from build123d import *

# Parameters (mm, degrees)
SKETCH_2_R          = 3
SKETCH_2_R_2        = 1.5
SKETCH_2_R_3        = 2.5
EXTRUDE_1_DEPTH     = 3
EXTRUDE_2_DEPTH     = 196
SKETCH_5_R          = 8
CUT_EXTRUDE_1_DEPTH = 10
SKETCH_6_R          = 4.05
CUT_EXTRUDE_2_DEPTH = 10
SKETCH_8_R          = 40
EXTRUDE_3_DEPTH     = 3
EXTRUDE_START       = -61
EXTRUDE_4_DEPTH     = 64
EXTRUDE_5_DEPTH     = 3
EXTRUDE_START_2     = -3
EXTRUDE_14_DEPTH    = 3
EXTRUDE_15_DEPTH    = 3
SKETCH_16_R         = 40
EXTRUDE_16_DEPTH    = 3
CUT_EXTRUDE_START   = -20
CUT_EXTRUDE_5_DEPTH = 20
CUT_EXTRUDE_6_DEPTH = 20
CUT_EXTRUDE_7_DEPTH = 3
FILLET_3_R          = 3
FILLET_4_R          = 3
FILLET_5_R          = 3
FILLET_6_R          = 3
SKETCH_22_R         = 7.75
CUT_EXTRUDE_8_DEPTH = 10
SKETCH_23_R         = 4.05
CUT_EXTRUDE_9_DEPTH = 10


# Some blends are built 0.0001 mm under size
with BuildPart() as part:
    # Sketch 2 → Extrude 1 (new body)
    with BuildSketch(Plane(origin=(0, 0, 0), x_dir=(0, 0, -1), z_dir=(1, 0, 0))):
        with BuildLine():
            Line((138.514809283, 84.200667909), (-11.70063651, 38.25042621))
            ThreePointArc((-11.70063651, 38.25042621), (-39.560188627, -5.915359313), (0, -40))
            Line((0, -40), (16.710190716, -40))
            Line((16.710190716, -40), (156.071648789, 40.329376559))
            Line((156.071648789, 40.329376559), (156.071648789, 43.792069046))
            ThreePointArc((156.071648789, 43.792069046), (165.334026038, 71.834783727), (138.514809283, 84.200667909))
        make_face()
        Circle(SKETCH_2_R, mode=Mode.SUBTRACT)
        with Locations((145, 70)):
            Circle(SKETCH_2_R_2, mode=Mode.SUBTRACT)
        with Locations((138, 63)):
            Circle(SKETCH_2_R_2, mode=Mode.SUBTRACT)
        with Locations((145, 56)):
            Circle(SKETCH_2_R_2, mode=Mode.SUBTRACT)
        with Locations((145, 63)):
            Circle(SKETCH_2_R_3, mode=Mode.SUBTRACT)
        with Locations((152, 63)):
            Circle(SKETCH_2_R_2, mode=Mode.SUBTRACT)
    extrude_1 = extrude(amount=EXTRUDE_1_DEPTH)

    # Sketch 4 → Extrude 2 (add)
    with BuildSketch(Plane(origin=(3, 0, 0), x_dir=(0, 0, -1), z_dir=(1, 0, 0))):
        with BuildLine():
            Line((0, -40), (16.710190716, -40))
            Line((16.710190716, -40), (156.071648789, 40.329376559))
            Line((156.071648789, 40.329376559), (156.071648789, 43.792069046))
            Line((156.071648789, 43.792069046), (19.975563357, -34.655113166))
            ThreePointArc((19.975563357, -34.655113166), (10.339136167, -38.640681455), (0, -40))
        make_face()
    extrude(amount=EXTRUDE_2_DEPTH)

    # Mirror 2: Extrude 1 across plane
    add(extrude_1.mirror(Plane(origin=(101, 0, 0), x_dir=(0, 0, 1), z_dir=(1, 0, 0))))

    # Sketch 5 → Cut-Extrude 1 (cut)
    with BuildSketch(Plane(origin=(202, 0, 0), x_dir=(0, 0, -1), z_dir=(1, 0, 0))):
        Circle(SKETCH_5_R)
    extrude(amount=-CUT_EXTRUDE_1_DEPTH, mode=Mode.SUBTRACT)

    # Sketch 6 → Cut-Extrude 2 (cut)
    with BuildSketch(Plane.ZY):
        Circle(SKETCH_6_R)
    extrude(amount=-CUT_EXTRUDE_2_DEPTH, mode=Mode.SUBTRACT)

    # Sketch 9 → Extrude 4 (add)
    with BuildSketch(Plane(origin=(251, 0, 0), x_dir=(0, 0, -1), z_dir=(1, 0, 0)).offset(EXTRUDE_START)):
        with BuildLine():
            Line((0, -40), (16.710190716, -40))
            Line((16.710190716, -40), (53.747942483, -18.651059269))
            Line((53.747942483, -18.651059269), (52.249775231, -16.051925781))
            Line((52.249775231, -16.051925781), (19.975563357, -34.655113166))
            ThreePointArc((19.975563357, -34.655113166), (10.339136167, -38.640681455), (0, -40))
        make_face()
    extrude_4 = extrude(amount=EXTRUDE_4_DEPTH)

    # Sketch 10 → Extrude 5 (add)
    with BuildSketch(Plane(origin=(0, -37.254246654, -21.473730609), x_dir=(1, 0, 0), z_dir=(0, -0.8663778291595938, -0.49938908392225567))):
        Polygon((254, -37.251890328), (254, -57.251890328), (202, -87.274104325), (202, -37.251890328), align=None)
    extrude_5 = extrude(amount=-EXTRUDE_5_DEPTH)



with BuildPart() as body_2:
    # Sketch 8 → Extrude 3 (new body)
    with BuildSketch(Plane(origin=(251, 0, 0), x_dir=(0, 0, -1), z_dir=(1, 0, 0))):
        Circle(SKETCH_8_R)
    extrude(amount=EXTRUDE_3_DEPTH)


with BuildPart() as part_1:
    add(part.part)

    add(body_2.part)  # Extrude 14 merges body 2
    # Sketch 14 → Extrude 14 (add)
    with BuildSketch(Plane(origin=(254, 0, 0), x_dir=(0, 0, -1), z_dir=(1, 0, 0)).offset(EXTRUDE_START_2)):
        with BuildLine():
            Line((-11.70063651, 38.25042621), (35.679778873, 52.743886101))
            Line((35.679778873, 52.743886101), (69.577331814, -6.064144103))
            Line((69.577331814, -6.064144103), (19.975563357, -34.655113166))
            ThreePointArc((19.975563357, -34.655113166), (36.686823541, 15.939792297), (-11.70063651, 38.25042621))
        make_face()
    extrude_14 = extrude(amount=EXTRUDE_14_DEPTH)

    # Sketch 15 → Extrude 15 (add)
    with BuildSketch(Plane(origin=(88.290795719, 76.368648195, -132.490087928), x_dir=(-0.8660254037844362, 0.24969454196113003, -0.4331889145798008), z_dir=(0.5000000000000044, 0.4324836330493111, -0.7503052093278204))):
        Polygon((-191.344507397, -43), (-191.344507397, 27.878041456), (-131.300079402, 20.97393325), (-131.300079402, -43), align=None)
    extrude_15 = extrude(amount=-EXTRUDE_15_DEPTH)

    # Mirror 8: Extrude 15 across plane
    add(extrude_15.mirror(Plane(origin=(101, 0, 0), x_dir=(0, 0, 1), z_dir=(1, 0, 0))))

    # Mirror 10: Extrude 5 across plane
    add(extrude_5.mirror(Plane(origin=(101, 0, 0), x_dir=(0, 0, 1), z_dir=(1, 0, 0))))

    # Mirror 11: Extrude 4 across plane
    add(extrude_4.mirror(Plane(origin=(101, 0, 0), x_dir=(0, 0, 1), z_dir=(1, 0, 0))))

    # Mirror 12: Extrude 14 across plane
    add(extrude_14.mirror(Plane(origin=(101, 0, 0), x_dir=(0, 0, 1), z_dir=(1, 0, 0))))

    # Sketch 16 → Extrude 16 (add)
    with BuildSketch(Plane.ZY.offset(52)):
        Circle(SKETCH_16_R)
    extrude(amount=-EXTRUDE_16_DEPTH)

    # Sketch 17 → Cut-Extrude 5 (cut)
    with BuildSketch(Plane(origin=(202, 0, 0), x_dir=(0, 0, -1), z_dir=(1, 0, 0)).offset(CUT_EXTRUDE_START)):
        with BuildLine():
            Line((-11.120326036, 38.423148607), (61.739147636, 60.715331959))
            Line((61.739147636, 60.715331959), (65.138195736, 61.755085767))
            Line((65.138195736, 61.755085767), (62.037518083, 60.197696416))
            Line((62.037518083, 60.197696416), (92.586691567, 7.198687311))
            Line((92.586691567, 7.198687311), (19.975563357, -34.655113166))
            ThreePointArc((19.975563357, -34.655113166), (-36.806411031, -15.66167638), (-11.120326036, 38.423148607))
        make_face()
    extrude(amount=CUT_EXTRUDE_5_DEPTH, mode=Mode.SUBTRACT)


with BuildPart() as cut_extrude_5_piece_1:
    # of the separate pieces the step leaves, piece 1, a body of its own (cut_extrude_5_pieces)
    add(part_1.part.solids().sort_by_distance((0, 43.792069046, -156.071648789))[0])

    # Sketch 21 → Cut-Extrude 7 (cut)
    with BuildSketch(Plane(origin=(3, 0, 0), x_dir=(0, 0, -1), z_dir=(1, 0, 0))):
        with BuildLine():
            Line((92.586691567, 7.198687311), (62.037518083, 60.197696416))
            Line((62.037518083, 60.197696416), (65.138195736, 61.755085767))
            Line((65.138195736, 61.755085767), (61.739147636, 60.715331959))
            Line((61.739147636, 60.715331959), (-11.70063651, 38.25042621))
            ThreePointArc((-11.70063651, 38.25042621), (-36.686823541, -15.939792297), (19.975563357, -34.655113166))
            Line((19.975563357, -34.655113166), (92.586691567, 7.198687311))
        make_face()
    extrude(amount=-CUT_EXTRUDE_7_DEPTH, mode=Mode.SUBTRACT)

    # Fillet 3
    fillet_3_edges = [cut_extrude_5_piece_1.edges().sort_by_distance(p)[0] for p in [
        (3, 33.698191863, -77.312104825),
    ]]
    fillet(fillet_3_edges, radius=FILLET_3_R - 0.0001)  # a hair under: the kernel refuses the full size

    # Fillet 4
    fillet_4_edges = [cut_extrude_5_piece_1.edges().sort_by_distance(p)[0] for p in [
        (199, 33.698191863, -77.312104825),
    ]]
    fillet(fillet_4_edges, radius=FILLET_4_R - 0.0001)  # a hair under: the kernel refuses the full size

    # Fillet 5
    # the kernel refuses this fillet: 3 mm, written as the material it adds along each edge
    with BuildSketch(Plane(origin=(202, 65.506611814, -62.97577757), x_dir=(0, 0.49938908392225534, -0.8663778291595939), z_dir=(0, -0.866377829159594, -0.4993890839222554))) as fillet_5_piece_1_section:
        with BuildLine():
            CenterArc((FILLET_5_R * 0.57735026919, FILLET_5_R), FILLET_5_R, 210, 60)
            Line((-FILLET_5_R * 0.288675134595, FILLET_5_R * 0.5), (0, 0))
            Line((0, 0), (FILLET_5_R * 0.57735026919, 0))
        make_face()
    fillet_5_piece_1 = extrude(amount=68.304060269, mode=Mode.PRIVATE)
    fillet_5_piece_1 = split(fillet_5_piece_1, bisect_by=Plane(origin=(202.325553984, 63.906694987, -72.171998522), z_dir=(0, -0.9562606552534866, -0.2925159127537726)), keep=Keep.TOP, mode=Mode.PRIVATE)
    fillet_5_piece_1 = split(fillet_5_piece_1, bisect_by=Plane(origin=(199.177617764, 62.412552566, -67.072312804), z_dir=(0.09892666816624712, -0.8892295154916122, -0.44663674625368427)), keep=Keep.TOP, mode=Mode.PRIVATE)
    add(fillet_5_piece_1)

    # Fillet 6
    # the kernel refuses this fillet: 3 mm, written as the material it adds along each edge
    with BuildSketch(Plane(origin=(0, 6.329488355, -97.086079656), x_dir=(2.017234182721707e-14, 0.49938908392225534, -0.8663778291595939), z_dir=(0, 0.8663778291595939, 0.4993890839222554))) as fillet_6_piece_1_section:
        with BuildLine():
            CenterArc((FILLET_6_R * 0.57735026919, FILLET_6_R), FILLET_6_R, 210, 60)
            Line((-FILLET_6_R * 0.288675134595, FILLET_6_R * 0.5), (0, 0))
            Line((0, 0), (FILLET_6_R * 0.57735026919, 0))
        make_face()
    fillet_6_piece_1 = extrude(amount=68.304060269, mode=Mode.PRIVATE)
    fillet_6_piece_1 = split(fillet_6_piece_1, bisect_by=Plane(origin=(-0.325553984, 63.906694987, -72.171998522), z_dir=(0, -0.9562606552534866, -0.2925159127537726)), keep=Keep.TOP, mode=Mode.PRIVATE)
    fillet_6_piece_1 = split(fillet_6_piece_1, bisect_by=Plane(origin=(2.822382236, 62.412552566, -67.072312804), z_dir=(-0.09892666816624712, -0.8892295154916122, -0.44663674625368427)), keep=Keep.TOP, mode=Mode.PRIVATE)
    add(fillet_6_piece_1)

    # Sketch 22 → Cut-Extrude 8 (cut)
    with BuildSketch(Plane(origin=(254, 0, 0), x_dir=(0, 0, -1), z_dir=(1, 0, 0))):
        Circle(SKETCH_22_R)
    extrude(amount=-CUT_EXTRUDE_8_DEPTH, mode=Mode.SUBTRACT)

    # Sketch 23 → Cut-Extrude 9 (cut)
    with BuildSketch(Plane.ZY.offset(52)):
        Circle(SKETCH_23_R)
    extrude(amount=-CUT_EXTRUDE_9_DEPTH, mode=Mode.SUBTRACT)


with BuildPart() as cut_extrude_5_piece_2:
    # of the separate pieces the step leaves, piece 2, a body of its own (cut_extrude_5_pieces)
    add(part_1.part.solids().sort_by_distance((202, 60.715331959, -61.739147636))[0])

    # Sketch 18 → Cut-Extrude 6 (cut)
    with BuildSketch(Plane(origin=(0, 38.25042621, 11.70063651), x_dir=(1, 0, 0), z_dir=(0, 0.9562606552534866, 0.2925159127537726))):
        Polygon((199, 76.798918519), (202, 76.932821805), (202, 0), (199, 0), align=None)
    extrude(amount=-CUT_EXTRUDE_6_DEPTH, mode=Mode.SUBTRACT)


solid = cut_extrude_5_piece_1.part
Build history of the part. All positions in model axes, mm. A direction names the side the tool comes from. Coordinates: 2 decimals unless noted, no trailing zeros. Order: outer loops, then holes, each group sorted by start corner. A loop starts at its lowest first (then second) coordinate and runs counter-clockwise, first axis right, second up. Notation, with made-up numbers: (-36.5, -22) -> (10.5, -22) arc R29 ccw to (10.5, 1) -> close; hole circle Ø1 at (30.25, 0). An arc over 180 degrees is marked (long way). One line per item, written item: value.
(1) Slice it at D-D, the plane y = -30.5. List the corners of the cut face in (x, z).
Checked values:
outline: (-52, -33.19) -> (254, -33.19) -> (254, 25.88) -> (251, 25.88) -> (251, -27.18) -> (-49, -27.18) -> (-49, 25.88) -> (-52, 25.88) -> close
(2) Slice it at A-A, the plane y = 77. List the corners of the cut face in (x, z).
Checked values:
outline: (0, -162.19) -> (3, -162.19) -> (3, -114.98) -> (0, -114.98) -> close; (199, -162.19) -> (202, -162.19) -> (202, -114.98) -> (199, -114.98) -> close
(3) Probe line 1 (X direction, y = -31, z = 18.5); line 2 (Y direction, x = 2.35, z = -145); line 3 (Y direction, x = 252.65, z = 0). List the from-to ranges inside material, lowest first. Write a range as [from, to].
Checked values:
line 1: [-52, -49], [251, 254]
line 2: [33.95, 54.5], [57.5, 60.5], [65.5, 68.5], [71.5, 85.17]
line 3: [-40, -7.75], [7.75, 41.83]
(4) Slice it at C-C, the plane z = 19.5. List the corners of the cut face in (x, y), plus the area to 3 significant figures.
Checked values:
outline: (-52, -34.92) -> (-49, -34.92) -> (-49, 34.92) -> (-52, 34.92) -> close; (251, -34.92) -> (254, -34.92) -> (254, 34.92) -> (251, 34.92) -> close
area: 419 mm2
(5) Drop flat-ended pins along their axis: pin 1 Ø2 at (x, z) = (211.5, -47.5) entering from +Y; pin 2 Ø1 at (x, y) = (133, 42) entering from -Z; pin 3 Ø6 at (x, y) = (109.5, -3.5) entering from -Z. Give the stop position or say it passes through.
Checked values:
pin 1: y = -18.21
pin 2: z = -156.07
pin 3: z = -85.24
(6) Tool access for faces 1 (the flat face through (199, 47, -115)), 2 (the flat face through (202, 47, -116)), 3 (the flat face through (0, 47, -116)), 4 (the cylindrical face through (199.855, 34.52, -77.88)): list every direction of +Z, -Z, +X, -X, +Y, -Y with a clear straight run to the whole face (end or side of a thin tool).
Checked values:
face 1: +Z, +Y
face 2: -Z, +X, +Y
face 3: -Z, -X, +Y
face 4: +Z
(7) Slice it at B-B, the plane x = 24.5. List the corners of the cut face in (y, z), plus the area to 3 significant figures.
Checked values:
outline: (-40, -16.71) -> (40.33, -156.07) -> (43.79, -156.07) -> (-34.66, -19.98) arc R40 cw to (-40, 0) -> close
area: 503 mm2
(8) Mould opens along Y. For faces 5 (the cylindrical face through (252.521, 7.684, 1.009)), 6 (the cylindrical face through (252.48, -5.13, 39.67)), 7 (the flat face through (-50.479, 45.396, -11.658)) say: pulls with the +Y half, pulls with the -Y half, needs draft (parallel to the pull), parting line crosses it, or undercut.
Checked values:
face 5: undercut
face 6: parting line crosses it
face 7: pulls with the +Y half
